```python
from build123d import *

# Parameters (mm, degrees)
F1_DEPTH = 100
F2_W     = 50
F2_H     = 15
F3_DEPTH = 74


with BuildPart() as f1:
    # F0 (on Front) → F1 (new body)
    with BuildSketch(Plane.XZ):
        Polygon((-15, 0), (0, 0), (0, 87), (74, 87), (74, 102), (-15, 102), align=None)
    extrude(amount=F1_DEPTH)

    # F2 (on face) → F3 (join)
    with BuildSketch(Plane.YZ):
        with Locations((-25, 7.5)):
            Rectangle(F2_W, F2_H)
    extrude(amount=F3_DEPTH)


solid = f1.part
```
Source: CAD feature listing. Evaluate the final solid. Frame: model axes, mm. A direction names the side the tool comes from. Round coordinates to 2 decimals unless told otherwise and drop trailing zeros. Loops run counter-clockwise (first coordinate to the right, second up) from the corner with the lowest first, then second, coordinate; pieces in that order, holes last. Notation, with made-up numbers: M 12.25,89.25 L 22.25,89.25 A6 cw 22.25,100.25 Z; hole C 60.5,-33 d2. An arc over 180 degrees is marked long. Use a Markdown table: item, result. Add a question column.
1. Ray query, line 1 along Z through (x, y) = (56, -16); line 2 along X through (y, z) = (-78.5, 63); line 3 along Y through (x, z) = (68.5, 14.5). Return the intervals inside material, ascending. Write a range as [from, to].
2. Cut plane B-B, the plane y = -7. Output: boundary loops of the cut face in (x, z).
3. Pull-direction query (Z, two-part tool) for faces 3 (the flat face through (30, -49, 102)), 4 (the flat face through (36, -50, 7)), 5 (the flat face through (0, -49, 43)); classes: +Z half, -Z half, draft (parallel to the pull), parting line (faces both ways), or undercut.
4. Cut plane D-D, the plane y = -93. Output: boundary loops of the cut face in (x, z), and give its area (3 significant figures).
5. Cut plane A-A, the plane x = 15. Output: boundary loops of the cut face in (y, z).
6. Set-up query: faces 1 (the flat face through (36, -49, 87)), 2 (the flat face through (74, -49, 94)). Return all of +Z, -Z, +X, -X, +Y, -Y with unobstructed straight access to the full face (end or side cutting, diameter ignored); none if empty.
7. Cut plane C-C, the plane z = 76. Output: boundary loops of the cut face in (x, y).
8. Contact query for a flat-ended pin moving along its axis: pin 1 (7.5 mm diameter, centred on x = 21, z = 4, fed in from -Y). Output: stop coordinate, or through.
Solution:
| question | item | result |
|---|---|---|
| 1 | line 1 | z = [0, 15], [87, 102] |
| 1 | line 2 | x = [-15, 0] |
| 1 | line 3 | y = [-50, 0] |
| 2 | outline | M -15,0 L 74,0 L 74,15 L 0,15 L 0,87 L 74,87 L 74,102 L -15,102 Z |
| 3 | face 3 | +Z half |
| 3 | face 4 | draft |
| 3 | face 5 | undercut |
| 4 | outline | M -15,0 L 0,0 L 0,87 L 74,87 L 74,102 L -15,102 Z |
| 4 | area | 2,640 mm2 |
| 5 | outline | M -100,87 L 0,87 L 0,102 L -100,102 Z; M -50,0 L 0,0 L 0,15 L -50,15 Z |
| 6 | face 1 | +X, +Y, -Y |
| 6 | face 2 | +Z, -Z, +X, +Y, -Y |
| 7 | outline | M -15,-100 L 0,-100 L 0,0 L -15,0 Z |
| 8 | pin 1 | stops at y = -50 |
